from build123d import *

# Parameters (mm, degrees)
SKETCH1_R           = 32
BOSS_EXTRUDE1_DEPTH = 10


with BuildPart() as part:
    # Sketch1 → Boss-Extrude1 (new body)
    # profile 1 of 2: a face of its own
    with BuildSketch(Plane(origin=(0, 0, 0), x_dir=(1, 0, 0), z_dir=(0, 1, 0))):
        with Locations((-186.104281586, 0)):
            Circle(SKETCH1_R)
        Polygon((-169.093123496, -0.251434953), (-180.608415791, 16.100875078), (-199.718807817, 10.202323), (-200.014387332, -9.7954927), (-181.086673492, -16.256270425), align=None, mode=Mode.SUBTRACT)
    # profile 2 of 2: a face of its own
    with BuildSketch(Plane(origin=(0, 0, 0), x_dir=(1, 0, 0), z_dir=(0, 1, 0))):
        with BuildLine():
            Line((0, 17), (-134, 17))
            Line((-134, 17), (-154.402546617, 17))
            ThreePointArc((-154.402546617, 17), (-158.25184177, 17.864711017), (-161.361464049, 20.292682927))
            ThreePointArc((-161.361464049, 20.292682927), (-155.973150167, 10.775663294), (-154.104281586, 0))
            ThreePointArc((-154.104281586, 0), (-155.973150167, -10.775663294), (-161.361464049, -20.292682927))
            ThreePointArc((-161.361464049, -20.292682927), (-158.25184177, -17.864711017), (-154.402546617, -17))
            Line((-154.402546617, -17), (-134, -17))
            Line((-134, -17), (0, -17))
            ThreePointArc((0, -17), (17, 0), (0, 17))
        make_face()
        with BuildLine():
            ThreePointArc((-134, -9), (-143, 0), (-134, 9))
            Line((-134, 9), (0, 9))
            ThreePointArc((0, 9), (9, 0), (0, -9))
            Line((0, -9), (-134, -9))
        make_face(mode=Mode.SUBTRACT)
    extrude(amount=BOSS_EXTRUDE1_DEPTH)


solid = part.part
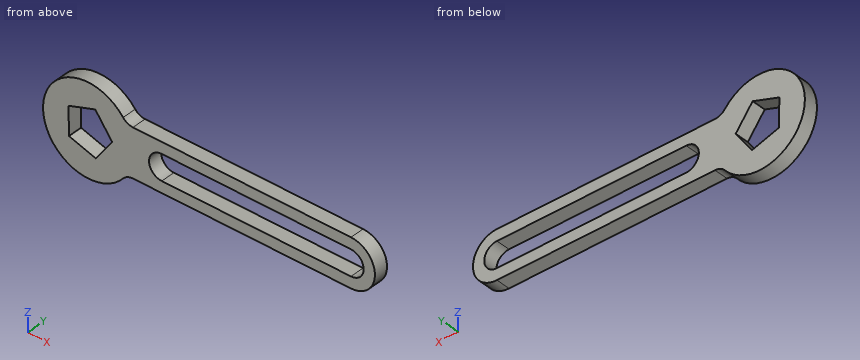
Check sheet for the modelled part. Datum: model origin and axes. Units: mm. Round coordinates to 2 decimals unless told otherwise and drop trailing zeros. Order: outer loops, then holes, each group sorted by start corner. A loop starts at its lowest first (then second) coordinate and runs counter-clockwise, first axis right, second up. Notation, with made-up numbers: M -32.5,48.25 L -15.5,48.25 A21 cw -15.5,65.25 Z; hole C 81.5,8 d9. An arc over 180 degrees is marked long. One line per item, written item: value. Start each with the question number.
1. Section check B-B on x = -52. Enter the section's corners in (y, z), and give its area (3 significant figures).
2. Section check D-D on z = 3.5. Enter the section's corners in (x, y).
3. Scan lines: line 1 along Z through (x, y) = (-74.5, 6.75); line 2 along X through (y, z) = (9.5, 8); line 3 along X through (y, z) = (3.25, 1). Record each from-to range of solid material in increasing order.
4. Gauge pin test, flat ends, axial feed: P1, Ø3, axis at y = 5, z = -9.5, coming from the -X side; P2, Ø5, axis at x = -36, y = 6.5, coming from the -Z side; P3, Ø3, axis at x = -65.5, y = 4.5, coming from the +Z side. Record the tip position at first contact, or that the pin passes through.
5. Section check C-C on z = -13.5. Enter the section's corners in (x, y).
6. Section check A-A on y = 4.25. Enter the section's corners in (x, z), and give its area (3 significant figures).
Results found:
1. outline: M 0,-17 L 10,-17 L 10,-9 L 0,-9 Z; M 0,9 L 10,9 L 10,17 L 0,17 Z
1. area: 160 mm^2
2. outline: M -217.91,0 L -199.92,0 L -199.92,10 L -217.91,10 Z; M -171.53,0 L -142.29,0 L -142.29,10 L -171.53,10 Z; M 8.29,0 L 16.64,0 L 16.64,10 L 8.29,10 Z
3. line 1: -17 to -9, 9 to 17
3. line 2: -217.09 to -199.99, -174.9 to -138.12, 4.12 to 15
3. line 3: -218.09 to -199.88, -169.65 to -142.94, 8.94 to 16.97
4. P1: x = -217.09
4. P2: z = -17
4. P3: z = 17
5. outline: M -215.12,0 L -189.03,0 L -189.03,10 L -215.12,10 Z; M -178.78,0 L 10.33,0 L 10.33,10 L -178.78,10 Z
6. outline: M -161.36,-20.29 A9 cw -154.4,-17 L 0,-17 A17 ccw 0,17 L -154.4,17 A9 cw -161.36,20.29 A32 ccw long Z; hole M -200.01,9.8 L -199.72,-10.2 L -180.61,-16.1 L -169.09,0.25 L -181.09,16.26 Z; hole M -134,-9 L 0,-9 A9 ccw 0,9 L -134,9 A9 ccw Z
6. area: 5,620 mm^2
